The model under review builds one solid part; all positions refer to its coordinate system, in mm. Face numbers are marked on the shaded views. A direction names the side the tool comes from. Coordinates: 2 decimals unless noted, no trailing zeros. Order: outer loops, then holes, each group sorted by start corner. A loop starts at its lowest first (then second) coordinate and runs counter-clockwise, first axis right, second up. Notation, with made-up numbers: M 86,-34.5 L 137,-34.5 A28 cw 137,2.5 Z; hole C 11,1 d11. An arc over 180 degrees is marked long. Answer in a Markdown table with one row per item.
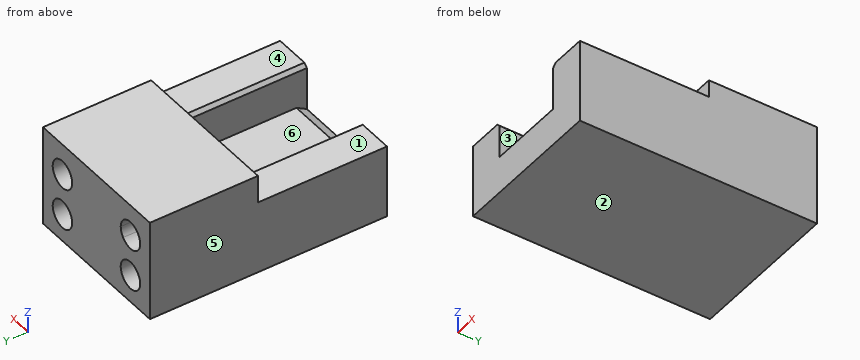
from build123d import *

# Parameters (mm, degrees)
F0_W     = 11
F0_H     = 1.5
F0_R     = 1.62
F0_R_2   = 2
F1_DEPTH = 15.5
F3_DEPTH = 18.5
F4_D     = 4
F4_DEPTH = 8
F4_TIP   = 1.2017212381
F5_DEPTH = 6
F6_SIZE2 = 0.8660254038
F6_SIZE  = 1.5


with BuildPart() as f1:
    # F0 (on Front) → F1 (new body)
    with BuildSketch(Plane.XZ):
        with Locations((-33.422443, -0.3)):
            Rectangle(F0_W, F0_H)
        with BuildLine():
            ThreePointArc((-42.3589346731, 3.25), (-41.3596463712, 0.9831808692), (-38.922443, 1.4271243445))
            Line((-38.922443, 1.4271243445), (-38.922443, 2.75))
            Line((-38.922443, 2.75), (-39.422443, 3.25))
            Line((-39.422443, 3.25), (-42.3589346731, 3.25))
        make_face()
        with BuildLine():
            Line((-38.922443, 1.4271243445), (-38.922443, 0.45))
            Line((-38.922443, 0.45), (-27.922443, 0.45))
            Line((-27.922443, 0.45), (-27.922443, 1.4271243445))
            Line((-27.922443, 1.4271243445), (-27.922443, 2.1381176584))
            ThreePointArc((-27.922443, 2.1381176584), (-28.042443, 2.75), (-27.922443, 3.3618823416))
            Line((-27.922443, 3.3618823416), (-27.922443, 4.25))
            Line((-27.922443, 4.25), (-27.422443, 4.75))
            Line((-27.422443, 4.75), (-26.4224430007, 4.75))
            Line((-26.4224430007, 4.75), (-22.422443, 4.75))
            Line((-22.422443, 4.75), (-22.422443, 7.25))
            Line((-22.422443, 7.25), (-44.422443, 7.25))
            Line((-44.422443, 7.25), (-44.422443, 3.25))
            Line((-44.422443, 3.25), (-42.3589346731, 3.25))
            ThreePointArc((-42.3589346731, 3.25), (-40.170434415, 4.7340593925), (-38.422443, 2.75))
            ThreePointArc((-38.422443, 2.75), (-38.5516143066, 2.0428932188), (-38.922443, 1.4271243445))
        make_face()
        with BuildLine():
            Line((-38.922443, 2.75), (-38.922443, 1.4271243445))
            ThreePointArc((-38.922443, 1.4271243445), (-38.5516143066, 2.0428932188), (-38.422443, 2.75))
            ThreePointArc((-38.422443, 2.75), (-40.170434415, 4.7340593925), (-42.3589346731, 3.25))
            Line((-42.3589346731, 3.25), (-39.422443, 3.25))
            Line((-39.422443, 3.25), (-38.922443, 2.75))
        make_face()
        with BuildLine():
            Line((-27.922443, 3.3618823416), (-27.922443, 2.1381176584))
            ThreePointArc((-27.922443, 2.1381176584), (-26.1106738546, 1.1602830441), (-24.802443, 2.75))
            ThreePointArc((-24.802443, 2.75), (-26.1106738546, 4.3397169559), (-27.922443, 3.3618823416))
        make_face()
        with BuildLine():
            Line((-27.922443, -1.05), (-38.922443, -1.05))
            Line((-38.922443, -1.05), (-38.922443, 0.45))
            Line((-38.922443, 0.45), (-38.922443, 1.4271243445))
            ThreePointArc((-38.922443, 1.4271243445), (-41.3596463712, 0.9831808692), (-42.3589346731, 3.25))
            Line((-42.3589346731, 3.25), (-44.422443, 3.25))
            Line((-44.422443, 3.25), (-44.422443, -7.25))
            Line((-44.422443, -7.25), (-22.422443, -7.25))
            Line((-22.422443, -7.25), (-22.422443, 4.75))
            Line((-22.422443, 4.75), (-26.4224430007, 4.75))
            ThreePointArc((-26.4224430007, 4.75), (-24.5995673443, 1.9271243448), (-27.922443, 1.4271243445))
            Line((-27.922443, 1.4271243445), (-27.922443, 0.45))
            Line((-27.922443, 0.45), (-27.922443, -1.05))
        make_face()
        with Locations((-40.422443, -3.25)):
            Circle(F0_R, mode=Mode.SUBTRACT)
        with Locations((-26.422443, -3.25)):
            Circle(F0_R_2, mode=Mode.SUBTRACT)
        with Locations((-26.422443, -3.25)):
            Circle(F0_R_2)
        with Locations((-40.422443, -3.25)):
            Circle(F0_R)
        with BuildLine():
            Line((-27.922443, 2.1381176584), (-27.922443, 1.4271243445))
            ThreePointArc((-27.922443, 1.4271243445), (-24.5995673443, 1.9271243448), (-26.4224430007, 4.75))
            Line((-26.4224430007, 4.75), (-27.422443, 4.75))
            Line((-27.422443, 4.75), (-27.922443, 4.25))
            Line((-27.922443, 4.25), (-27.922443, 3.3618823416))
            ThreePointArc((-27.922443, 3.3618823416), (-26.1106738546, 4.3397169559), (-24.802443, 2.75))
            ThreePointArc((-24.802443, 2.75), (-26.1106738546, 1.1602830441), (-27.922443, 2.1381176584))
        make_face()
        with BuildLine():
            ThreePointArc((-27.922443, 3.3618823416), (-28.042443, 2.75), (-27.922443, 2.1381176584))
            Line((-27.922443, 2.1381176584), (-27.922443, 3.3618823416))
        make_face()
    extrude(amount=F1_DEPTH)

    # F2 (on face) → F3 (join)
    with BuildSketch(Plane.XZ.offset(15.5)):
        Polygon((-27.922443, -1.05), (-38.922443, -1.05), (-38.922443, 2.75), (-39.422443, 3.25), (-44.422443, 3.25), (-44.422443, -7.25), (-22.422443, -7.25), (-22.422443, 4.75), (-27.422443, 4.75), (-27.922443, 4.25), align=None)
    extrude(amount=F3_DEPTH)

    # F4
    with Locations(Plane(origin=(0, 0, 0), x_dir=(1, 0, 0), z_dir=(0, 1, 0))):
        with Locations((-40.422443, 3.25), (-26.422443, -2.75)):
            Hole(F4_D / 2, depth=F4_DEPTH)
            with Locations((0, 0, -(F4_DEPTH + F4_TIP / 2))):  # 118° drill point
                Cone(0, F4_D / 2, F4_TIP, mode=Mode.SUBTRACT)

    # F0 (on Front) → F5 (cut)
    with BuildSketch(Plane.XZ):
        with BuildLine():
            Line((-38.922443, 2.75), (-38.922443, 1.4271243445))
            ThreePointArc((-38.922443, 1.4271243445), (-38.5516143066, 2.0428932188), (-38.422443, 2.75))
            ThreePointArc((-38.422443, 2.75), (-40.170434415, 4.7340593925), (-42.3589346731, 3.25))
            Line((-42.3589346731, 3.25), (-39.422443, 3.25))
            Line((-39.422443, 3.25), (-38.922443, 2.75))
        make_face()
        with BuildLine():
            ThreePointArc((-42.3589346731, 3.25), (-41.3596463712, 0.9831808692), (-38.922443, 1.4271243445))
            Line((-38.922443, 1.4271243445), (-38.922443, 2.75))
            Line((-38.922443, 2.75), (-39.422443, 3.25))
            Line((-39.422443, 3.25), (-42.3589346731, 3.25))
        make_face()
        with Locations((-26.422443, -3.25)):
            Circle(F0_R_2)
    extrude(amount=F5_DEPTH, mode=Mode.SUBTRACT)

    # F6
    f6_edges = [f1.edges().sort_by_distance(p)[0] for p in [
        (-33.422443, -34, -1.05),
    ]]
    f6_side = f1.faces().sort_by_distance((-33.422443, -24.75, -1.05))[0]
    chamfer(f6_edges, length=F6_SIZE, length2=F6_SIZE2, reference=f6_side)


solid = f1.part
(1) Machinability: for the marked faces 1, 2 and 3, which of the approach directions +Z, -Z, +X, -X, +Y, -Y give a long, thin tool a straight path to every point of the face, cutting with its end or side? Answer none if there is none.
Report:
| item | result |
|---|---|
| face 1 | +Z, -X, -Y |
| face 2 | -Z, +X, -X, +Y, -Y |
| face 3 | +Z, -Y |
(2) Insertion check: P1, Ø1.5, axis at x = -42, y = -24.5, coming from the +Z side; P2, Ø2.5, axis at x = -26.42, z = 2.75, coming from the +Y side; P3, Ø2, axis at x = -26, z = -2.5, coming from the +Y side. Each pin has a flat end and moves straight along its axis. Give the tip position at first contact, or say it passes through.
Report:
| item | result |
|---|---|
| P1 | z = 3.25 |
| P2 | y = -8.45 |
| P3 | y = -6 |
(3) Take a section at A-A (y = -23.5). Write out the cut boundary in (x, z), then the cut area to 3 significant figures.
Report:
| item | result |
|---|---|
| outline | M -44.42,-7.25 L -22.42,-7.25 L -22.42,4.75 L -27.42,4.75 L -27.92,4.25 L -27.92,-1.05 L -38.92,-1.05 L -38.92,2.75 L -39.42,3.25 L -44.42,3.25 Z |
| area | 192 mm^2 |
(4) Take a section at B-B (x = -30.25). Write out the cut boundary in (y, z).
Report:
| item | result |
|---|---|
| outline | M -34,-7.25 L 0,-7.25 L 0,7.25 L -15.5,7.25 L -15.5,-1.05 L -32.5,-1.05 L -34,-1.92 Z |
(5) The part is to be moulded in two halves that separate along X. For the marked faces 4, 5 and 6, say which applies: +X half, -X half, draft (parallel to the pull), parting line (faces both ways), or undercut.
Report:
| item | result |
|---|---|
| face 4 | draft |
| face 5 | -X half |
| face 6 | undercut |
(6) To check wall thickness, follow line 1 (X direction, y = -5, z = 4.25); line 2 (X direction, y = -3.5, z = 3); line 3 (Z direction, x = -33.5, y = -24.5). State the ranges of each line that lie inside material, in increasing order. Write a range as [from, to].
Report:
| item | result |
|---|---|
| line 1 | [-44.42, -41.75], [-39.1, -27.75], [-25.1, -22.42] |
| line 2 | [-44.42, -42.41], [-38.44, -28.41], [-24.44, -22.42] |
| line 3 | [-7.25, -1.05] |
